Source: CAD feature listing. Evaluate the final solid. Frame: model axes, mm. Round coordinates to 2 decimals unless told otherwise and drop trailing zeros. Write each loop counter-clockwise with the first axis right and the second up, starting at its lowest first coordinate (ties: lowest second). Pieces come first, ordered by that corner, then holes. Notation, with made-up numbers: M 34,-38 L 67,-38 A17 ccw 67,-7 Z; hole C 16,69.25 d7. An arc over 180 degrees is marked long. Use a Markdown table: item, result.
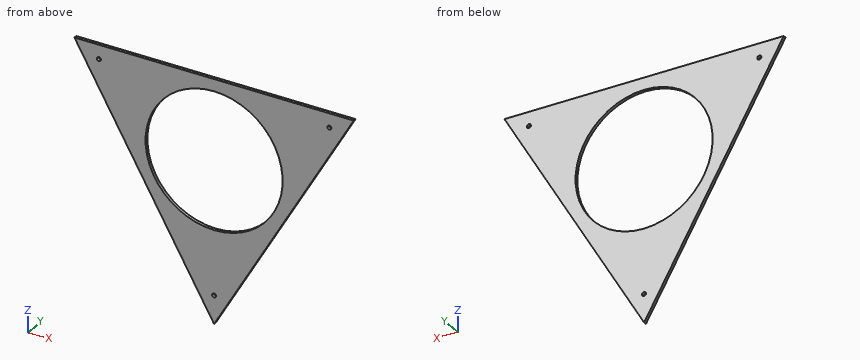
```python
from build123d import *

# Parameters (mm, degrees)
BOSS_EXTRUDE1_DEPTH     = 4.7625
CUT_EXTRUDE3_DEPTH      = 4.7625
CUT_EXTRUDE3_DEPTH_BACK = 4.7625
SKETCH5_R               = 107.95
SKETCH6_R               = 3.175
CUT_EXTRUDE5_DEPTH      = 4.7625


with BuildPart() as part:
    # Sketch1 → Boss-Extrude1 (new body)
    with BuildSketch(Plane(origin=(0, 0, 0), x_dir=(1, 0, 0), z_dir=(0, 1, 0))):
        Polygon((0, 254), (-219.970452561, -127), (219.970452561, -127), align=None)
    extrude(amount=BOSS_EXTRUDE1_DEPTH)

    # Sketch5 → Cut-Extrude3 (cut, two sides: drawn at the far end of the back side and taken through both)
    with BuildSketch(Plane(origin=(0, 0, 0), x_dir=(1, 0, 0), z_dir=(0, 1, 0)).offset(-CUT_EXTRUDE3_DEPTH_BACK)):
        with Locations(Location((0, 0, 0), (0, 0, 90))):
            Circle(SKETCH5_R)
    extrude(amount=CUT_EXTRUDE3_DEPTH + CUT_EXTRUDE3_DEPTH_BACK, mode=Mode.SUBTRACT)

    # Sketch6 → Cut-Extrude5 (cut)
    with BuildSketch(Plane(origin=(0, 0, 0), x_dir=(1, 0, 0), z_dir=(0, 1, 0))):
        with Locations(Location((-181.475623363, -104.775, 0), (0, 0, 90))):
            Circle(SKETCH6_R)
        with Locations(Location((0, 209.55, 0), (0, 0, 90))):
            Circle(SKETCH6_R)
    cut_extrude5 = extrude(amount=CUT_EXTRUDE5_DEPTH, mode=Mode.SUBTRACT)

    # Mirror1: Cut-Extrude5 across plane
    add(cut_extrude5.mirror(Plane(origin=(0, 0, 0), x_dir=(0, 0, 1), z_dir=(1, 0, 0))), mode=Mode.SUBTRACT)


solid = part.part
```
Q1. Line query: L1, parallel to Z at x = -81.5, y = 2.35; L2, parallel to Z at x = 7, y = 1.9; L3, parallel to X at y = 4.3, z = -21. Output: solid intervals per line, ascending.
Results are:
| item | result |
|---|---|
| L1 | -112.84 to -70.79, 70.79 to 127 |
| L2 | -241.88 to -107.72, 107.72 to 127 |
| L3 | -134.52 to -105.89, 105.89 to 134.52 |
Q2. First-contact query: pin 1 Ø1 at (y, z) = (2.5, -175.5) entering from -X. Flat tip, straight axial feed; report the tip coordinate or a pass-through.
Results are:
| item | result |
|---|---|
| pin 1 | x = -45.61 |
Q3. Section A-A on z = 0. Return loops of the section in (x, y), plus the area to 3 significant figures.
Results are:
| item | result |
|---|---|
| outline | M -146.65,0 L -107.95,0 L -107.95,4.76 L -146.65,4.76 Z; M 107.95,0 L 146.65,0 L 146.65,4.76 L 107.95,4.76 Z |
| area | 369 mm^2 |
Q4. Section D-D on x = -166. Return loops of the section in (y, z), plus the area to 3 significant figures.
Results are:
| item | result |
|---|---|
| outline | M 0,33.52 L 4.76,33.52 L 4.76,127 L 0,127 Z |
| area | 445 mm^2 |
Q5. Section C-C on y = 3.1. Return loops of the section in (x, z) (3 decimals), plus the area to 3 significant figures.
Results are:
| item | result |
|---|---|
| outline | M -219.97,127 L 0,-254 L 219.97,127 Z; hole C -181.476,104.775 d6.35; hole C 0,0 d215.9; hole C 0,-209.55 d6.35; hole C 181.476,104.775 d6.35 |
| area | 47,100 mm^2 |
Q6. Section B-B on x = -36. Return loops of the section in (y, z).
Results are:
| item | result |
|---|---|
| outline | M 0,-191.65 L 4.76,-191.65 L 4.76,-101.77 L 0,-101.77 Z; M 0,101.77 L 4.76,101.77 L 4.76,127 L 0,127 Z |
